For this review, take the finished solid that the model builds, in its own axes (mm). A direction names the side the tool comes from. Give positions to 0.01 mm unless a question says otherwise; leave off trailing zeros. Order: outer loops, then holes, each group sorted by start corner. A loop starts at its lowest first (then second) coordinate and runs counter-clockwise, first axis right, second up. Notation, with made-up numbers: M 58.5,62.5 L 71.5,62.5 A29 ccw 71.5,86.5 Z; hole C 45,18 d2. An arc over 180 degrees is marked long. Use CSV: the item, a comma, the result in double quotes. Start each with the question number.
(1) Tool access review of faces 1 (the face through (1, 9.239, 2)), 2 (the face through (2.2, 11.739, 3.3)): name each direction out of +Z, -Z, +X, -X, +Y, -Y from which nothing blocks a thin tool from reaching the whole face with its end or side.
(2) Consider section A-A (z = 0). Write out the cut boundary in (x, y).
(3) Draft analysis for pull direction X (two halves, no side actions). For faces 3 (the face through (-0.715, 11.211, 1.375)), 4 (the face through (0, 13.239, 0)), 5 (the face through (-3.233, 10.506, 1.341)), 6 (the face through (0, 14.239, 0)), state which applies: pulls with the +X half, pulls with the -X half, needs draft (parallel to the pull), parting line crosses it, or undercut.
(4) Consider section D-D (y = 12.65). Write out the cut boundary in (x, z), and give its area (3 significant figures).
(5) Clearance check with flat-ended pins moving along their axes: P1, Ø2, axis at y = 13.5, z = 4, coming from the -X side; P2, Ø2, axis at y = 11, z = 1, coming from the +X side; P3, Ø3, axis at x = -1, y = 13.5, coming from the -Z side; P4, Ø2, axis at x = -3.5, z = 1, coming from the -Y side. State where each tip first meets the part, or that it passes through.
(6) Wall thickness on L1, parallel to X at y = 11.35, z = 0; L2, parallel to Z at x = 0, y = 11.9: over which ranges is each line inside the solid? List them lowest first. Write a range as from..to.
(7) Consider section C-C (y = 10.3). Write out the cut boundary in (x, z), and give its area (3 significant figures).
(8) Consider section B-B (x = 0). Write out the cut boundary in (y, z).
```python
from build123d import *


with BuildPart() as part:
    # Esboço1 → Revolução1 (revolve)
    with BuildSketch(Plane.XY):
        with BuildLine():
            Line((-1.55, 9.238932358), (-3.5, 9.238932358))
            Line((-3.5, 9.238932358), (-3.5, 11.738932358))
            Line((-3.5, 11.738932358), (-5, 11.738932358))
            Line((-5, 11.738932358), (-5, 11.838932358))
            ThreePointArc((-5, 11.838932358), (-4.297056275, 13.535988633), (-2.6, 14.238932358))
            Line((-2.6, 14.238932358), (0, 14.238932358))
            Line((0, 14.238932358), (0, 13.238932358))
            Line((0, 13.238932358), (-1.55, 13.238932358))
            Line((-1.55, 13.238932358), (-1.55, 9.238932358))
        make_face()
    revolve(axis=Axis((0, 36.954647584, 0), (0, -1, 0)))


solid = part.part
```
Check result:
1,face 1,"+Z, -Z, +X, -X, -Y"
1,face 2,"-Y"
2,outline,"M -5,11.74 L -3.5,11.74 L -3.5,9.24 L -1.55,9.24 L -1.55,13.24 L 1.55,13.24 L 1.55,9.24 L 3.5,9.24 L 3.5,11.74 L 5,11.74 L 5,11.84 A2.4 ccw 2.6,14.24 L -2.6,14.24 A2.4 ccw -5,11.84 Z"
3,face 3,"undercut"
3,face 4,"undercut"
3,face 5,"parting line crosses it"
3,face 6,"needs draft"
4,outline,"C 0,0 d9.72; hole C 0,0 d3.1"
4,area,"66.6 mm^2"
5,P1,"stops at x = -3.51"
5,P2,"stops at x = 4.99"
5,P3,"stops at z = -4.97"
5,P4,"stops at y = 9.24"
6,L1,"x = -3.5..-1.55, 1.55..3.5"
6,L2,"z = -5..-1.55, 1.55..5"
7,outline,"C 0,0 d7; hole C 0,0 d3.1"
7,area,"30.9 mm^2"
8,outline,"M 9.24,-3.5 L 11.74,-3.5 L 11.74,-5 L 11.84,-5 A2.4 ccw 14.24,-2.6 L 14.24,2.6 A2.4 ccw 11.84,5 L 11.74,5 L 11.74,3.5 L 9.24,3.5 L 9.24,1.55 L 13.24,1.55 L 13.24,-1.55 L 9.24,-1.55 Z"
